Autodesk Inventor part; units mm, degrees
ref_plane "YZ Plane" through (0, 0, 0) normal (1, 0, 0) x (0, 1, 0)
ref_plane "XZ Plane" through (0, 0, 0) normal (0, 1, 0) x (-1, 0, 0)
ref_plane "XY Plane" through (0, 0, 0) normal (0, 0, 1) x (1, 0, 0)
sketch "Sketch1" plane through (0, 0, 0) normal (0, 1, 0) x (-1, 0, 0)
  line L0 (0, 0) -> (127, 0)
  line L1 (127, 0) -> (127, 76.2)
  line L2 (127, 76.2) -> (0, 76.2)
  line L3 (0, 76.2) -> (0, 0)
  dimension "d0" = 127
  dimension "d2" = 76.2
extrude "Extrusion1" add sketch "Sketch1" along normal blind 3.175
sketch "Sketch2" plane through (0, 0, 0) normal (0, -1, 0) x (1, 0, 0)
  line L0 (0, 0) -> (-127, 0)
  line L1 (0, 76.2) -> (0, 0)
  line L2 (-127, 76.2) -> (0, 76.2)
  line L3 (-127, 0) -> (-127, 76.2)
  point P0 (-114.3, 63.5)
  point P1 (-12.7, 63.5)
  point P2 (-12.7, 12.7)
  point P3 (-114.3, 12.7)
  dimension "d5" = 12.7
  dimension "d6" = 12.7
  dimension "d7" = 12.7
  dimension "d8" = 12.7
  dimension "d9" = 12.7
  dimension "d10" = 12.7
  dimension "d11" = 12.7
  dimension "d12" = 12.7
hole "Hole1" at (-114.3, 0, 63.5) at (-12.7, 0, 63.5) at (-12.7, 0, 12.7) at (-114.3, 0, 12.7) direction (0, 1, 0) diameter 6.35 end through all
sketch "Sketch3" plane through (0, 3.175, 0) normal (0, 1, 0) x (1, 0, 0)
  line L0 (-127, -76.2) -> (0, -76.2)
  line L1 (0, -76.2) -> (0, 0)
  line L2 (0, 0) -> (-127, 0)
  point P0 (-38.1, -63.5)
  point P1 (-38.1, -12.7)
  dimension "d20" = 12.7
  dimension "d21" = 38.1
  dimension "d29" = 12.7
  dimension "d30" = 38.1
hole "Hole2" at (-38.1, 3.175, 63.5) at (-38.1, 3.175, 12.7) direction (0, -1, 0) diameter 6.35 end through all
properties part number "MountSwitchBar" material "Aluminum 6061"
CAD build for the part. Positions are in the model's coordinates, mm. Round coordinates to 2 decimals unless told otherwise and drop trailing zeros. Order: outer loops, then holes, each group sorted by start corner. A loop starts at its lowest first (then second) coordinate and runs counter-clockwise, first axis right, second up. Notation, with made-up numbers: (-33, -36) -> (-1, -36) arc R27 ccw to (-1, -20) -> close; hole circle Ø8 at (2.25, 46.5). An arc over 180 degrees is marked (long way). Write each question's results on one line, items separated by ' | '.
1. Wall check: line 1 along X through (y, z) = (1.65, 63.5) (3 decimals); line 2 along Z through (x, y) = (-38.1, 1.15) (3 decimals); line 3 along X through (y, z) = (0.95, 14). Give the ranges that are in metal, low to high. Write a range as [from, to].
Findings below:
line 1: x = [-127, -117.475], [-111.125, -41.275], [-34.925, -15.875], [-9.525, 0] | line 2: z = [0, 9.525], [15.875, 60.325], [66.675, 76.2] | line 3: x = [-127, -117.2], [-111.4, -41], [-35.2, -15.6], [-9.8, 0]
2. Pull direction X, two halves, no side cores. Call faces 1 (the face through (0, 2, 39)), 2 (the face through (-39.05, 1.57, 66.53)), 3 (the face through (-63, 2, 0)), 4 (the face through (-11.48, 1.61, 60.57)): pulls with the +X half, pulls with the -X half, needs draft (parallel to the pull), parting line crosses it, or undercut.
Findings below:
face 1: pulls with the +X half | face 2: undercut | face 3: needs draft | face 4: undercut
3. Flat gauge pin, fed straight in: P1, Ø5, axis at x = -114.3, z = 63.5, coming from the +Y side. Where does the tip first touch, or does it go through?
Findings below:
P1: passes through
4. Cut at B-B (x = -114.3). Give the cut face in (y, z) (3 decimals), plus the area to 3 significant figures.
Findings below:
outline: (0, 0) -> (3.175, 0) -> (3.175, 9.525) -> (0, 9.525) -> close; (0, 15.875) -> (3.175, 15.875) -> (3.175, 60.325) -> (0, 60.325) -> close; (0, 66.675) -> (3.175, 66.675) -> (3.175, 76.2) -> (0, 76.2) -> close | area: 202 mm²
5. Cut at A-A (z = 12.7). Give the cut face in (x, y) (3 decimals), plus the area to 3 significant figures.
Findings below:
outline: (-127, 0) -> (-117.475, 0) -> (-117.475, 3.175) -> (-127, 3.175) -> close; (-111.125, 0) -> (-41.275, 0) -> (-41.275, 3.175) -> (-111.125, 3.175) -> close; (-34.925, 0) -> (-15.875, 0) -> (-15.875, 3.175) -> (-34.925, 3.175) -> close; (-9.525, 0) -> (0, 0) -> (0, 3.175) -> (-9.525, 3.175) -> close | area: 343 mm²
6. Cut at C-C (y = 1.75). Give the cut face in (x, z) (3 decimals).
Findings below:
outline: (-127, 0) -> (0, 0) -> (0, 76.2) -> (-127, 76.2) -> close; hole circle Ø6.35 at (-114.3, 12.7); hole circle Ø6.35 at (-114.3, 63.5); hole circle Ø6.35 at (-38.1, 12.7); hole circle Ø6.35 at (-38.1, 63.5); hole circle Ø6.35 at (-12.7, 12.7); hole circle Ø6.35 at (-12.7, 63.5)
